```python
from build123d import *

# Parameters (mm, degrees)
SKETCH1_W           = 29.5
SKETCH1_H           = 12.5
BOSS_EXTRUDE1_DEPTH = 5
SKETCH2_W           = 10
SKETCH2_H           = 8
CUT_EXTRUDE1_DEPTH  = 6
FILLET1_R           = 2
FILLET2_R           = 1.5
SKETCH3_W           = 21.5
SKETCH3_H           = 5
CUT_EXTRUDE2_DEPTH  = 2


with BuildPart() as part:
    # Sketch1 → Boss-Extrude1 (new body)
    with BuildSketch(Plane(origin=(0, 0, 0), x_dir=(1, 0, 0), z_dir=(0, 1, 0))):
        Rectangle(SKETCH1_W, SKETCH1_H)
    extrude(amount=BOSS_EXTRUDE1_DEPTH)

    # Sketch2 → Cut-Extrude1 (cut, through all)
    with BuildSketch(Plane(origin=(0, 5, 0), x_dir=(1, 0, 0), z_dir=(0, 1, 0))):
        with Locations((0, -2.25)):
            Rectangle(SKETCH2_W, SKETCH2_H)
    extrude(amount=-CUT_EXTRUDE1_DEPTH, mode=Mode.SUBTRACT)

    # Fillet1
    fillet1_edges = [part.edges().sort_by_distance(p)[0] for p in [
        (-14.75, 2.5, -6.25),
        (14.75, 2.5, -6.25),
    ]]
    fillet(fillet1_edges, radius=FILLET1_R)

    # Fillet2
    fillet2_edges = [part.edges().sort_by_distance(p)[0] for p in [
        (-5, 2.5, -1.75),
        (5, 2.5, -1.75),
    ]]
    fillet(fillet2_edges, radius=FILLET2_R)

    # Sketch3 → Cut-Extrude2 (cut)
    with BuildSketch(Plane.XY.offset(6.25)):
        with Locations((0, 2.5)):
            Rectangle(SKETCH3_W, SKETCH3_H)
    extrude(amount=-CUT_EXTRUDE2_DEPTH, mode=Mode.SUBTRACT)


solid = part.part
```
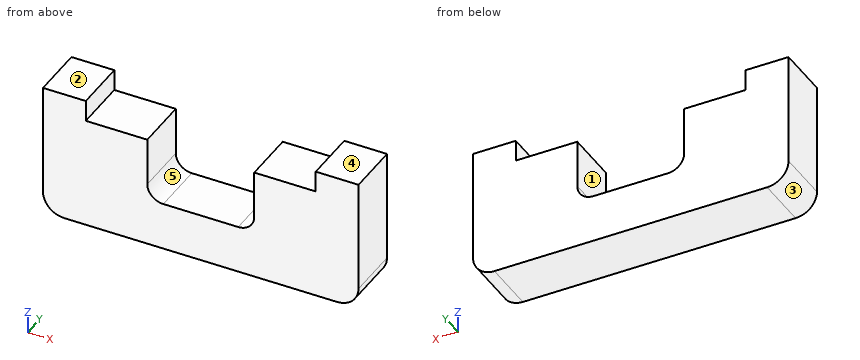
Source: CAD feature listing. Evaluate the final solid. Frame: model axes, mm. Face numbers are marked on the shaded views. A direction names the side the tool comes from. Round coordinates to 2 decimals unless told otherwise and drop trailing zeros. Loops run counter-clockwise (first coordinate to the right, second up) from the corner with the lowest first, then second, coordinate; pieces in that order, holes last.
(1) Contact query for flat-ended pins moving along their axis: pin 1 Ø2.5 at (x, y) = (7, 2) entering from +Z; pin 2 Ø2.5 at (x, y) = (0, 3.5) entering from +Z. Output: stop coordinate, or through.
From the geometry:
pin 1: stops at z = 4.25
pin 2: stops at z = -1.75
(2) Pull-direction query (X, two-part tool) for the marked faces 3, 4 and 5; classes: +X half, -X half, draft (parallel to the pull), parting line (faces both ways), or undercut.
From the geometry:
face 3: -X half
face 4: draft
face 5: undercut
(3) Section query A-A (z = 5.25). Output: boundary loops of the cut face in (x, y).
From the geometry:
outline: (-14.75, 0) - (-10.75, 0) - (-10.75, 5) - (-14.75, 5) - close; (10.75, 0) - (14.75, 0) - (14.75, 5) - (10.75, 5) - close
(4) Material intervals for probe 1 along X at (y, z) = (0.4, 2); probe 2 along X at (y, z) = (4.6, 5); probe 3 along Z at (x, y) = (-3.5, 1.85), sorted ascending.
From the geometry:
probe 1: x = -14.75 to -5, 5 to 14.75
probe 2: x = -14.75 to -10.75, 10.75 to 14.75
probe 3: z = -6.25 to -1.75
(5) Section query D-D (x = -2). Output: boundary loops of the cut face in (y, z), and give its area (3 significant figures).
From the geometry:
outline: (0, -6.25) - (5, -6.25) - (5, -1.75) - (0, -1.75) - close
area: 22.5 mm2
(6) Access query for the marked faces 1 and 2. Directions: +Z, -Z, +X, -X, +Y, -Y. A direction counts if a zero-diameter tool reaches every point of the face in a straight line with its end or side. Return the directions, or none.
From the geometry:
face 1: +Z, +Y, -Y
face 2: +Z, +X, -X, +Y, -Y
(7) Section query B-B (y = 2.3). Output: boundary loops of the cut face in (x, z), and give its area (3 significant figures).
From the geometry:
outline: (-14.75, -4.25) arc R2 ccw to (-12.75, -6.25) - (12.75, -6.25) arc R2 ccw to (14.75, -4.25) - (14.75, 6.25) - (10.75, 6.25) - (10.75, 4.25) - (5, 4.25) - (5, -0.25) arc R1.5 cw to (3.5, -1.75) - (-3.5, -1.75) arc R1.5 cw to (-5, -0.25) - (-5, 4.25) - (-10.75, 4.25) - (-10.75, 6.25) - (-14.75, 6.25) - close
area: 265 mm2
(8) Section query C-C (z = -0.75). Output: boundary loops of the cut face in (x, y).
From the geometry:
outline: (-14.75, 0) - (-4.91, 0) - (-4.91, 5) - (-14.75, 5) - close; (4.91, 0) - (14.75, 0) - (14.75, 5) - (4.91, 5) - close
